Part model, mm, in its own coordinate system. A direction names the side the tool comes from. Round coordinates to 2 decimals unless told otherwise and drop trailing zeros. Write each loop counter-clockwise with the first axis right and the second up, starting at its lowest first coordinate (ties: lowest second). Pieces come first, ordered by that corner, then holes. Notation, with made-up numbers: M -37.75,3.5 L 2.25,3.5 A18 ccw 2.25,16.5 Z; hole C -16,59 d10. An arc over 180 degrees is marked long. Use a Markdown table: item, result. Add a question column.
1) Slice it at B-B on z = 0. Write the cut outline in (x, y), plus the area to 3 significant figures.
2) Slice it at A-A on x = 24.5. Write the cut outline in (y, z) (3 decimals), plus the area to 3 significant figures.
3) Which spindle directions (+Z, -Z, +X, -X, +Y, -Y) get a long thin tool onto all of the face, cutting with end or side? Do faces 1 (the face through (18.561, 1, -25)), 2 (the face through (-12.238, 1, 41)), 3 (the face through (41, 1, 12.238)). Say none if no direction does.
4) Two-plate mould, pull along Z, no slides. Class faces 4 (the face through (18.561, 1, 24)), 5 (the face through (-43, 2, -7.738)), 6 (the face through (0, 1, 54.9)), 7 (the face through (12.238, 1, -41)): released by +Z, released by -Z, zero draft, split by the parting line, or undercut.
5) Wall check: probe 1 along Z at (x, y) = (-23, 1.65) (3 decimals); probe 2 along Z at (x, y) = (44, 0.4). Give the ranges that are in metal, low to high.
6) Drop flat-ended pins along their axis: P1, Ø5, axis at x = 40.15, z = 0, coming from the +Y side; P2, Ø1.5, axis at x = 43, y = 1, coming from the -Z side; P3, Ø1.5, axis at y = 2, z = -44.5, coming from the -X side; P4, Ø1.5, axis at x = -44, y = 1, coming from the -Z side. Give the stop position or say it passes through.
7) Slice it at C-C on y = 2.25. Give the number of separate pieces and of enclosed holes in the cut face, plus the area to 3 significant figures.
```python
from build123d import *

# Parameters (mm, degrees)
SKETCH1_R           = 1.5
BOSS_EXTRUDE1_DEPTH = 3
SKETCH2_R           = 1
SKETCH2_R_2         = 5
CUT_EXTRUDE1_DEPTH  = 3
SKETCH3_W           = 5
SKETCH3_H           = 3
SKETCH3_W_2         = 3
SKETCH3_H_2         = 5
CUT_EXTRUDE3_DEPTH  = 3


with BuildPart() as part:
    # Sketch1 → Boss-Extrude1 (new body)
    with BuildSketch(Plane(origin=(0, 0, 0), x_dir=(1, 0, 0), z_dir=(0, 1, 0))):
        with BuildLine():
            Line((36.795388519, -12.237658296), (44.9, -12.237658296))
            ThreePointArc((44.9, -12.237658296), (51.971067812, -9.308726108), (54.9, -2.237658296))
            Line((54.9, -2.237658296), (54.9, 3.1))
            ThreePointArc((54.9, 3.1), (51.971067812, 10.171067812), (44.9, 13.1))
            Line((44.9, 13.1), (36.795388519, 13.1))
            ThreePointArc((36.795388519, 13.1), (36.232963903, 13.332963903), (36, 13.895388519))
            Line((36, 13.895388519), (36, 32))
            ThreePointArc((36, 32), (34.828427125, 34.828427125), (32, 36))
            Line((32, 36), (13.033046814, 36))
            ThreePointArc((13.033046814, 36), (12.470622199, 36.232963903), (12.237658296, 36.795388519))
            Line((12.237658296, 36.795388519), (12.237658296, 44.9))
            ThreePointArc((12.237658296, 44.9), (9.308726108, 51.971067812), (2.237658296, 54.9))
            Line((2.237658296, 54.9), (-3.1, 54.9))
            ThreePointArc((-3.1, 54.9), (-10.171067812, 51.971067812), (-13.1, 44.9))
            Line((-13.1, 44.9), (-13.1, 36.795388519))
            ThreePointArc((-13.1, 36.795388519), (-13.332963903, 36.232963903), (-13.895388519, 36))
            Line((-13.895388519, 36), (-32, 36))
            ThreePointArc((-32, 36), (-34.828427125, 34.828427125), (-36, 32))
            Line((-36, 32), (-36, 13.033046814))
            ThreePointArc((-36, 13.033046814), (-36.232963903, 12.470622199), (-36.795388519, 12.237658296))
            Line((-36.795388519, 12.237658296), (-44.9, 12.237658296))
            ThreePointArc((-44.9, 12.237658296), (-51.971067812, 9.308726108), (-54.9, 2.237658296))
            Line((-54.9, 2.237658296), (-54.9, -3.1))
            ThreePointArc((-54.9, -3.1), (-51.971067812, -10.171067812), (-44.9, -13.1))
            Line((-44.9, -13.1), (-36.795388519, -13.1))
            ThreePointArc((-36.795388519, -13.1), (-36.232963903, -13.332963903), (-36, -13.895388519))
            Line((-36, -13.895388519), (-36, -32))
            ThreePointArc((-36, -32), (-34.828427125, -34.828427125), (-32, -36))
            Line((-32, -36), (-13.033046814, -36))
            ThreePointArc((-13.033046814, -36), (-12.470622199, -36.232963903), (-12.237658296, -36.795388519))
            Line((-12.237658296, -36.795388519), (-12.237658296, -44.9))
            ThreePointArc((-12.237658296, -44.9), (-9.308726108, -51.971067812), (-2.237658296, -54.9))
            Line((-2.237658296, -54.9), (3.1, -54.9))
            ThreePointArc((3.1, -54.9), (10.171067812, -51.971067812), (13.1, -44.9))
            Line((13.1, -44.9), (13.1, -36.795388519))
            ThreePointArc((13.1, -36.795388519), (13.332963903, -36.232963903), (13.895388519, -36))
            Line((13.895388519, -36), (32, -36))
            ThreePointArc((32, -36), (34.828427125, -34.828427125), (36, -32))
            Line((36, -32), (36, -13.033046814))
            ThreePointArc((36, -13.033046814), (36.232963903, -12.470622199), (36.795388519, -12.237658296))
        make_face()
        with Locations(Location((40.15, 0, 0), (0, 0, 270))):
            Circle(SKETCH1_R, mode=Mode.SUBTRACT)
        with Locations(Location((0, -40.15, 0), (0, 0, 270))):
            Circle(SKETCH1_R, mode=Mode.SUBTRACT)
        with Locations(Location((-40.15, 0, 0), (0, 0, 270))):
            Circle(SKETCH1_R, mode=Mode.SUBTRACT)
        with Locations(Location((0, 40.15, 0), (0, 0, 270))):
            Circle(SKETCH1_R, mode=Mode.SUBTRACT)
        with BuildLine():
            Line((20.560920379, 18.560920379), (28.535, 18.560920379))
            ThreePointArc((28.535, 18.560920379), (29.949213562, 19.146706817), (30.535, 20.560920379))
            Line((30.535, 20.560920379), (30.535, 28.535))
            ThreePointArc((30.535, 28.535), (29.949213562, 29.949213562), (28.535, 30.535))
            Line((28.535, 30.535), (20.560920379, 30.535))
            ThreePointArc((20.560920379, 30.535), (19.146706817, 29.949213562), (18.560920379, 28.535))
            Line((18.560920379, 28.535), (18.560920379, 20.560920379))
            ThreePointArc((18.560920379, 20.560920379), (19.146706817, 19.146706817), (20.560920379, 18.560920379))
        make_face(mode=Mode.SUBTRACT)
        with BuildLine():
            Line((4, -6), (-4, -6))
            ThreePointArc((-4, -6), (-5.414213562, -5.414213562), (-6, -4))
            Line((-6, -4), (-6, 4))
            ThreePointArc((-6, 4), (-5.414213562, 5.414213562), (-4, 6))
            Line((-4, 6), (4, 6))
            ThreePointArc((4, 6), (5.414213562, 5.414213562), (6, 4))
            Line((6, 4), (6, -4))
            ThreePointArc((6, -4), (5.414213562, -5.414213562), (4, -6))
        make_face(mode=Mode.SUBTRACT)
        with BuildLine():
            Line((-20.560920379, 18.560920379), (-28.535, 18.560920379))
            ThreePointArc((-28.535, 18.560920379), (-29.949213562, 19.146706817), (-30.535, 20.560920379))
            Line((-30.535, 20.560920379), (-30.535, 28.535))
            ThreePointArc((-30.535, 28.535), (-29.949213562, 29.949213562), (-28.535, 30.535))
            Line((-28.535, 30.535), (-20.560920379, 30.535))
            ThreePointArc((-20.560920379, 30.535), (-19.146706817, 29.949213562), (-18.560920379, 28.535))
            Line((-18.560920379, 28.535), (-18.560920379, 20.560920379))
            ThreePointArc((-18.560920379, 20.560920379), (-19.146706817, 19.146706817), (-20.560920379, 18.560920379))
        make_face(mode=Mode.SUBTRACT)
        with BuildLine():
            Line((18.560920379, -20.560920379), (18.560920379, -28.535))
            ThreePointArc((18.560920379, -28.535), (19.146706817, -29.949213562), (20.560920379, -30.535))
            Line((20.560920379, -30.535), (28.535, -30.535))
            ThreePointArc((28.535, -30.535), (29.949213562, -29.949213562), (30.535, -28.535))
            Line((30.535, -28.535), (30.535, -20.560920379))
            ThreePointArc((30.535, -20.560920379), (29.949213562, -19.146706817), (28.535, -18.560920379))
            Line((28.535, -18.560920379), (20.560920379, -18.560920379))
            ThreePointArc((20.560920379, -18.560920379), (19.146706817, -19.146706817), (18.560920379, -20.560920379))
        make_face(mode=Mode.SUBTRACT)
        with BuildLine():
            Line((-20.560920379, -18.560920379), (-28.535, -18.560920379))
            ThreePointArc((-28.535, -18.560920379), (-29.949213562, -19.146706817), (-30.535, -20.560920379))
            Line((-30.535, -20.560920379), (-30.535, -28.535))
            ThreePointArc((-30.535, -28.535), (-29.949213562, -29.949213562), (-28.535, -30.535))
            Line((-28.535, -30.535), (-20.560920379, -30.535))
            ThreePointArc((-20.560920379, -30.535), (-19.146706817, -29.949213562), (-18.560920379, -28.535))
            Line((-18.560920379, -28.535), (-18.560920379, -20.560920379))
            ThreePointArc((-18.560920379, -20.560920379), (-19.146706817, -19.146706817), (-20.560920379, -18.560920379))
        make_face(mode=Mode.SUBTRACT)
    extrude(amount=BOSS_EXTRUDE1_DEPTH)

    # Sketch2 → Cut-Extrude1 (cut)
    with BuildSketch(Plane(origin=(0, 3, 0), x_dir=(1, 0, 0), z_dir=(0, 1, 0))):
        with Locations(Location((-14.5, -32, 0), (0, 0, 270))):
            Circle(SKETCH2_R)
        with Locations(Location((0.5, -32, 0), (0, 0, 270))):
            Circle(SKETCH2_R)
        with Locations(Location((-14.5, 8, 0), (0, 0, 270))):
            Circle(SKETCH2_R)
        with Locations(Location((0.5, 8, 0), (0, 0, 270))):
            Circle(SKETCH2_R)
        with Locations(Location((0.5, -22.947694259, 0), (0, 0, 270))):
            Circle(SKETCH2_R_2)
        with Locations(Location((-22.947694259, -0.5, 0), (0, 0, 270))):
            Circle(SKETCH2_R_2)
        with Locations(Location((-0.5, 22.947694259, 0), (0, 0, 270))):
            Circle(SKETCH2_R_2)
        with Locations(Location((22.947694259, 0.5, 0), (0, 0, 270))):
            Circle(SKETCH2_R_2)
    extrude(amount=-CUT_EXTRUDE1_DEPTH, mode=Mode.SUBTRACT)

    # Sketch3 → Cut-Extrude3 (cut)
    with BuildSketch(Plane(origin=(0, 3, 0), x_dir=(1, 0, 0), z_dir=(0, 1, 0))):
        with Locations((-43.4, 9.237658296)):
            Rectangle(SKETCH3_W, SKETCH3_H)
        with Locations((-43.4, -9.237658296)):
            Rectangle(SKETCH3_W, SKETCH3_H)
        with Locations((9.237658296, 43.4)):
            Rectangle(SKETCH3_W_2, SKETCH3_H_2)
        with Locations((-9.237658296, 43.4)):
            Rectangle(SKETCH3_W_2, SKETCH3_H_2)
        with Locations((43.4, -9.237658296)):
            Rectangle(SKETCH3_W, SKETCH3_H)
        with Locations((43.4, 9.237658296)):
            Rectangle(SKETCH3_W, SKETCH3_H)
        with Locations((-9.237658296, -43.4)):
            Rectangle(SKETCH3_W_2, SKETCH3_H_2)
        with Locations((9.237658296, -43.4)):
            Rectangle(SKETCH3_W_2, SKETCH3_H_2)
    extrude(amount=-CUT_EXTRUDE3_DEPTH, mode=Mode.SUBTRACT)


solid = part.part
```
Entries:
| question | item | result |
|---|---|---|
| 1 | outline | M -54.9,0 L -41.65,0 L -41.65,3 L -54.9,3 Z; M -38.65,0 L -27.92,0 L -27.92,3 L -38.65,3 Z; M -17.97,0 L -6,0 L -6,3 L -17.97,3 Z; M 6,0 L 17.97,0 L 17.97,3 L 6,3 Z; M 27.92,0 L 38.65,0 L 38.65,3 L 27.92,3 Z; M 41.65,0 L 54.9,0 L 54.9,3 L 41.65,3 Z |
| 1 | area | 216 mm^2 |
| 2 | outline | M 0,-36 L 3,-36 L 3,-30.535 L 0,-30.535 Z; M 0,-18.561 L 3,-18.561 L 3,-5.253 L 0,-5.253 Z; M 0,4.253 L 3,4.253 L 3,18.561 L 0,18.561 Z; M 0,30.535 L 3,30.535 L 3,36 L 0,36 Z |
| 2 | area | 116 mm^2 |
| 3 | face 1 | +Y, -Y |
| 3 | face 2 | +Z, -X, +Y, -Y |
| 3 | face 3 | +Z, +X, +Y, -Y |
| 4 | face 4 | undercut |
| 4 | face 5 | undercut |
| 4 | face 6 | released by +Z |
| 4 | face 7 | zero draft |
| 5 | probe 1 | z = -36 to -30.535, -18.561 to -4.5, 5.5 to 18.561, 30.535 to 36 |
| 5 | probe 2 | z = -13.1 to -10.74, -7.74 to 7.74, 10.74 to 12.24 |
| 6 | P1 | stops at y = 3 |
| 6 | P2 | stops at z = -13.1 |
| 6 | P3 | stops at x = -13.1 |
| 6 | P4 | stops at z = -12.24 |
| 7 | separate pieces | 1 |
| 7 | enclosed holes | 25 |
| 7 | area | 5,740 mm^2 |
